Geometry check sheet. Reference: drawing and pictorial views, mm from the part's lowest x, y, z. Round coordinates to 2 decimals unless told otherwise and drop trailing zeros. Write each loop counter-clockwise with the first axis right and the second up, starting at its lowest first coordinate (ties: lowest second). Pieces come first, ordered by that corner, then holes. Notation, with made-up numbers: M 0,-16.75 L 24,-16.75 A17 cw 24,11.25 Z; hole C -27,32 d5. An arc over 180 degrees is marked long. Use a Markdown table: item, result. Add a question column.
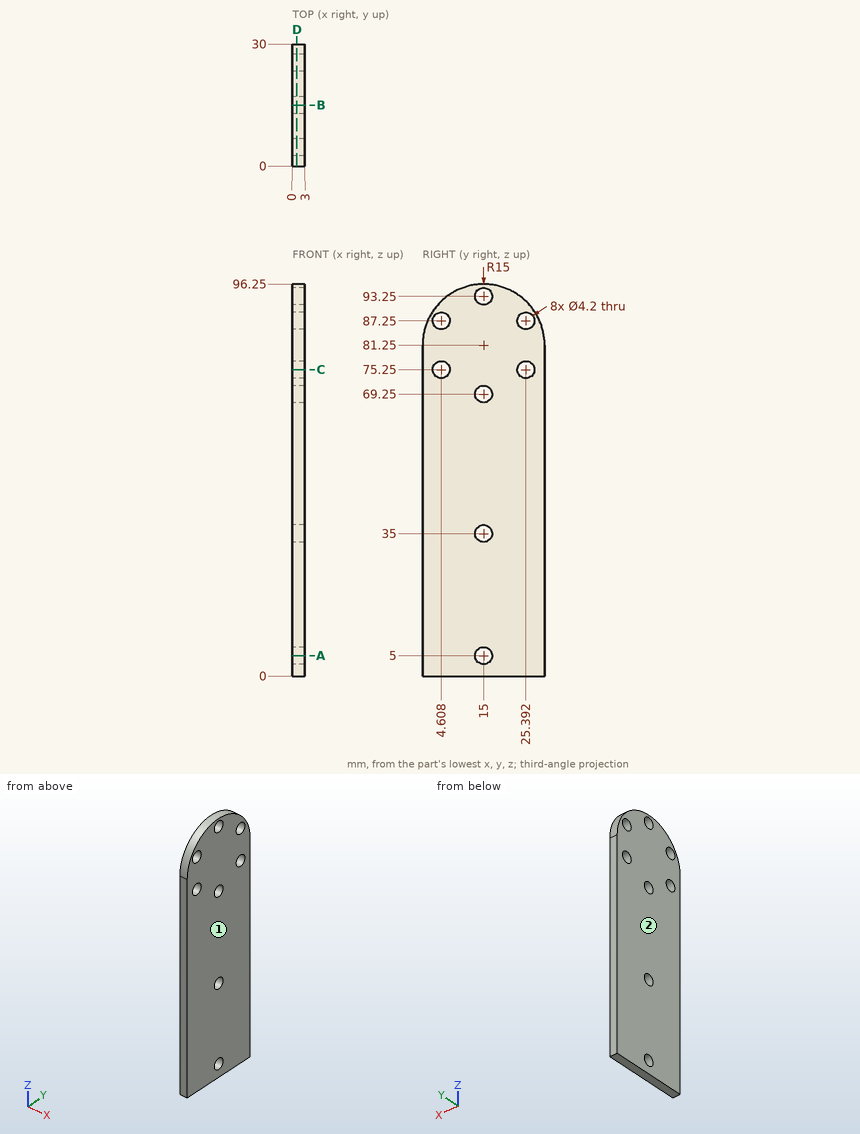
1. Cross-section at C-C on z = 75.25. Enter the section's corners in (x, y).
2. Release check for a two-part mould opening along X. For the marked faces 1 and 2 record: +X half, -X half, draft (parallel to the pull), parting line (faces both ways), or undercut.
3. Cross-section at A-A on z = 5. Enter the section's corners in (x, y).
4. Depth check by flat-ended pin: pin 1 Ø3.5 at (y, z) = (15, 5) entering from -X. Enter the tip coordinate at first touch or a pass-through.
5. Cross-section at B-B on y = 15. Enter the section's corners in (x, z), plus the area to 3 significant figures.
6. Scan lines: line 1 along Z through (x, y) = (1.45, 15.25) (1 decimal); line 2 along Y through (x, z) = (1.9, 75.25); line 3 along Y through (x, z) = (1, 35). Record each from-to range of solid material in increasing order. Write a range as from..to.
7. Cross-section at D-D on x = 1.1. Count the separate pieces of the cut face and the enclosed holes in it, plus the area to 3 significant figures.
Answer:
| question | item | result |
|---|---|---|
| 1 | outline | M 0,0 L 3,0 L 3,2.51 L 0,2.51 Z; M 0,6.71 L 3,6.71 L 3,23.29 L 0,23.29 Z; M 0,27.49 L 3,27.49 L 3,30 L 0,30 Z |
| 2 | face 1 | +X half |
| 2 | face 2 | -X half |
| 3 | outline | M 0,0 L 3,0 L 3,12.9 L 0,12.9 Z; M 0,17.1 L 3,17.1 L 3,30 L 0,30 Z |
| 4 | pin 1 | passes through |
| 5 | outline | M 0,0 L 3,0 L 3,2.9 L 0,2.9 Z; M 0,7.1 L 3,7.1 L 3,32.9 L 0,32.9 Z; M 0,37.1 L 3,37.1 L 3,67.15 L 0,67.15 Z; M 0,71.35 L 3,71.35 L 3,91.15 L 0,91.15 Z; M 0,95.35 L 3,95.35 L 3,96.25 L 0,96.25 Z |
| 5 | area | 238 mm^2 |
| 6 | line 1 | z = 0..2.9, 7.1..32.9, 37.1..67.2, 71.3..91.2, 95.3..96.2 |
| 6 | line 2 | y = 0..2.51, 6.71..23.29, 27.49..30 |
| 6 | line 3 | y = 0..12.9, 17.1..30 |
| 7 | separate pieces | 1 |
| 7 | enclosed holes | 8 |
| 7 | area | 2,680 mm^2 |
